Study the drawing (mm; zero at the part's minimum x, y, z) and answer. A direction names the side the tool comes from. Give positions to 0.01 mm unless a question says otherwise; leave off trailing zeros. Write each loop counter-clockwise with the first axis right and the second up, starting at its lowest first coordinate (ties: lowest second). Pieces come first, ordered by that corner, then holes. Notation, with made-up numbers: (83, 56.5) - (102, 56.5) arc R13 ccw to (102, 63.5) - close; hole circle Ø1 at (56.5, 84.5). An arc over 180 degrees is marked (long way). One line per item, written item: value. Start each with the question number.
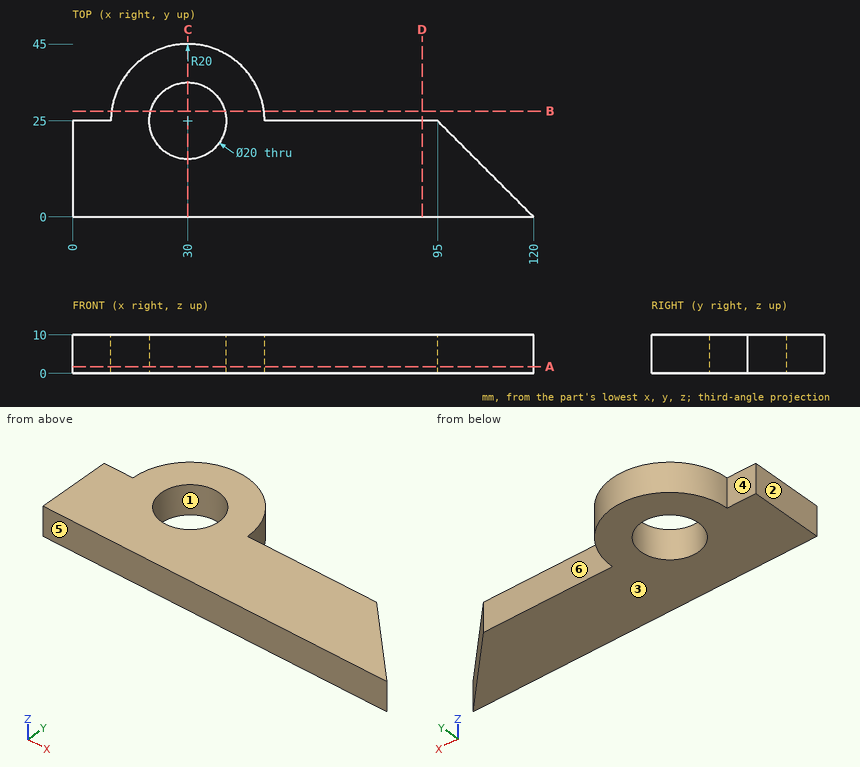
Item 1: Find section B-B on y = 27.5. Determine the outline of the cut face in (x, z), plus the area to 3 significant figures.
Item 2: Find section D-D on x = 91. Determine the outline of the cut face in (y, z).
Item 3: For the marked faces 4, 5 and 6, determine the directions among +Z, -Z, +X, -X, +Y, -Y from which every point of the face is accessible in a straight line to the end or side of a thin tool.
Item 4: Find section A-A on z = 1.75. Determine the outline of the cut face in (x, y).
Item 5: Each of these flat-tipped pins is pushed along its axis until it touches: pin 1 Ø5 at (y, z) = (38.5, 8.5) entering from -X; pin 2 Ø1 at (x, z) = (34, 6) entering from -Y; pin 3 Ø3 at (x, z) = (6, 3.5) entering from +Y. Where does it stop, or does it pass through?
Item 6: Straight lines are drawn through the part: line 1 along Y through (x, z) = (30, 2); line 2 along Y through (x, z) = (65, 9.25); line 3 along X through (y, z) = (16, 7.5). For each, find the intervals that lie inside material, in ascending order.
Item 7: The mould has two halves that part along X. Classify the marked faces 1, 2 and 3: +X half, -X half, draft (parallel to the pull), parting line (faces both ways), or undercut.
Item 8: Find section C-C on x = 30. Determine the outline of the cut face in (y, z), plus the area to 3 significant figures.
Values:
1. outline: (10.16, 0) - (20.32, 0) - (20.32, 10) - (10.16, 10) - close; (39.68, 0) - (49.84, 0) - (49.84, 10) - (39.68, 10) - close
1. area: 203 mm^2
2. outline: (0, 0) - (25, 0) - (25, 10) - (0, 10) - close
3. face 4: +Z, -Z, -X, +Y
3. face 5: +Z, -Z, +X, -X, -Y
3. face 6: +Z, -Z, +X, +Y
4. outline: (0, 0) - (120, 0) - (95, 25) - (50, 25) arc R20 ccw to (10, 25) - (0, 25) - close; hole circle Ø20 at (30, 25)
5. pin 1: x = 13.3
5. pin 2: y = 0
5. pin 3: y = 25
6. line 1: 0 to 15, 35 to 45
6. line 2: 0 to 25
6. line 3: 0 to 25.64, 34.36 to 104
7. face 1: undercut
7. face 2: -X half
7. face 3: draft
8. outline: (0, 0) - (15, 0) - (15, 10) - (0, 10) - close; (35, 0) - (45, 0) - (45, 10) - (35, 10) - close
8. area: 250 mm^2
